Source: CAD feature listing. Evaluate the final solid. Frame: model axes, mm. Face numbers are marked on the shaded views. A direction names the side the tool comes from. Coordinates: 2 decimals unless noted, no trailing zeros. Order: outer loops, then holes, each group sorted by start corner. A loop starts at its lowest first (then second) coordinate and runs counter-clockwise, first axis right, second up. Notation, with made-up numbers: (35, 78) -> (84, 78) arc R15 cw to (84, 89) -> close; hole circle Ø3 at (-28, 15.5). An arc over 180 degrees is marked (long way). Put each result on its own line as item: value.
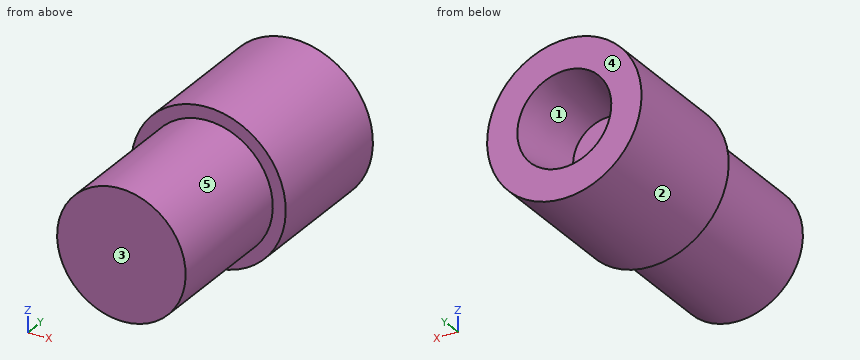
from build123d import *

# Parameters (mm, degrees)
SKETCH2_R          = 2.5
CUT_EXTRUDE1_DEPTH = 5
DRAFT1_ANGLE       = 10


with BuildPart() as part:
    # Sketch1 → Revolve1 (revolve)
    with BuildSketch(Plane.XY, mode=Mode.PRIVATE) as revolve1_sk:
        Polygon((0, 20), (5.55625, 20), (5.55625, 10), (4.625, 10), (4.625, 0), (0, 0), align=None)
    revolve(revolve1_sk.sketch.rotate(Axis((0, 0, 0), (0, 1, 0)), 90), axis=Axis((0, 0, 0), (0, 1, 0)))

    # Sketch2 → Cut-Extrude1 (cut)
    with BuildSketch(Plane(origin=(0, 20, 0), x_dir=(1, 0, 0), z_dir=(0, 1, 0))):
        with Locations(Location((0, 0, 0), (0, 0, 270))):
            Circle(SKETCH2_R)
    extrude(amount=-CUT_EXTRUDE1_DEPTH, mode=Mode.SUBTRACT)

    # Draft1
    draft1_faces = [part.faces().sort_by_distance(p)[0] for p in [
        (0, 17.5, -2.5),
    ]]
    draft(draft1_faces, Plane.ZX.offset(15), DRAFT1_ANGLE)


solid = part.part
1. Pull-direction query (X, two-part tool) for the marked faces 1, 2 and 3; classes: pulls with the +X half, pulls with the -X half, needs draft (parallel to the pull), parting line crosses it, or undercut.
Numbers:
face 1: undercut
face 2: parting line crosses it
face 3: needs draft
2. First-contact query: pin 1 (2 mm diameter, centred on x = -1, z = -0.5, fed in from +Y); pin 2 (1 mm diameter, centred on y = 16.5, z = 1, fed in from -X); pin 3 (3 mm diameter, centred on x = -2.5, y = 8, fed in from -Z). Flat tips, straight axial feed; report the tip coordinate or a pass-through.
Numbers:
pin 1: stops at y = 15
pin 2: stops at x = -5.53
pin 3: stops at z = -4.52
3. Set-up query: the marked faces 4 and 5. Return all of +Z, -Z, +X, -X, +Y, -Y with unobstructed straight access to the full face (end or side cutting, diameter ignored); none if empty.
Numbers:
face 4: +Z, -Z, +X, -X, +Y
face 5: -Y
4. Ray query, line 1 along Y through (x, z) = (3.75, -3); line 2 along X through (y, z) = (19.25, 2.5); line 3 along Y through (x, z) = (-1.5, -1). Return the intervals inside material, ascending.
Numbers:
line 1: y = 10 to 20
line 2: x = -4.96 to -2.08, 2.08 to 4.96
line 3: y = 0 to 15
5. Cut plane D-D on y = 15.5. Output: boundary loops of the cut face in (x, z), plus the area to 3 significant figures.
Numbers:
outline: circle Ø11.11 at (0, 0); hole circle Ø5.18 at (0, 0)
area: 75.9 mm2
6. Cut plane A-A on x = 0. Output: boundary loops of the cut face in (y, z) (3 decimals), plus the area to 3 significant figures.
Numbers:
outline: (0, -4.625) -> (10, -4.625) -> (10, -5.556) -> (20, -5.556) -> (20, -3.382) -> (15, -2.5) -> (15, 2.5) -> (20, 3.382) -> (20, 5.556) -> (10, 5.556) -> (10, 4.625) -> (0, 4.625) -> close
area: 174 mm2
7. Cut plane B-B on z = 0. Output: boundary loops of the cut face in (x, y) (3 decimals).
Numbers:
outline: (-5.556, 10) -> (-4.625, 10) -> (-4.625, 0) -> (4.625, 0) -> (4.625, 10) -> (5.556, 10) -> (5.556, 20) -> (3.382, 20) -> (2.5, 15) -> (-2.5, 15) -> (-3.382, 20) -> (-5.556, 20) -> close
8. Cut plane C-C on y = 13.25. Output: boundary loops of the cut face in (x, z).
Numbers:
outline: circle Ø11.11 at (0, 0)
